from build123d import *

# Parameters (mm, degrees)
SKETCH1_W           = 54.8
SKETCH1_H           = 59.3
BOSS_EXTRUDE1_DEPTH = 3
FILLET1_R           = 2.2
SKETCH2_W           = 3
SKETCH2_H           = 15
CUT_EXTRUDE1_DEPTH  = 41.483113764
CUT_EXTRUDE2_DEPTH  = 1.5


with BuildPart() as part:
    # Sketch1 → Boss-Extrude1 (new body)
    with BuildSketch(Plane(origin=(0, 0, 0), x_dir=(1, 0, 0), z_dir=(0, 1, 0))):
        Rectangle(SKETCH1_W, SKETCH1_H)
    extrude(amount=BOSS_EXTRUDE1_DEPTH)

    # Fillet1
    fillet1_edges = [part.edges().sort_by_distance(p)[0] for p in [
        (27.4, 1.5, 29.65),
        (-27.4, 1.5, 29.65),
        (-27.4, 1.5, -29.65),
        (27.4, 1.5, -29.65),
    ]]
    fillet(fillet1_edges, radius=FILLET1_R)

    # Sketch2 → Cut-Extrude1 (cut, through all)
    with BuildSketch(Plane(origin=(0, 3, 0), x_dir=(1, 0, 0), z_dir=(0, 1, 0))):
        with Locations((-24.5, -8.5)):
            Rectangle(SKETCH2_W, SKETCH2_H)
    extrude(amount=-CUT_EXTRUDE1_DEPTH, mode=Mode.SUBTRACT)

    # Sketch2<3> → Cut-Extrude2 (cut)
    with BuildSketch(Plane(origin=(0, 3, 0), x_dir=(1, 0, 0), z_dir=(0, 1, 0))):
        Polygon((-26, -16), (-26, -26), (26, -26), (26, 2), (-26, 2), (-26, -1), (-23, -1), (-23, -16), align=None)
    extrude(amount=-CUT_EXTRUDE2_DEPTH, mode=Mode.SUBTRACT)


solid = part.part
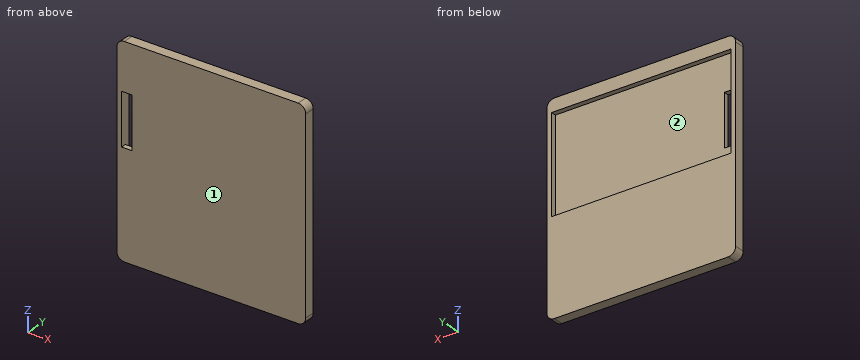
Input: part model. Units: mm. Frame: model coordinates. Face numbers are marked on the shaded views. Coordinates: 2 decimals unless noted, no trailing zeros. Loops run counter-clockwise (first coordinate to the right, second up) from the corner with the lowest first, then second, coordinate; pieces in that order, holes last. Notation, with made-up numbers: (-27.75, -35.75) -> (-16.75, -35.75) arc R21 cw to (-16.75, 0.25) -> close; hole circle Ø3 at (-33.5, 72.5). An arc over 180 degrees is marked (long way). Write item = value, one per line. Start each with the question number.
Item 1: Cut plane C-C, the plane x = -10.5. Return loops of the section in (y, z), plus the area to 3 significant figures.
Item 2: Cut plane B-B, the plane z = 9.5. Return loops of the section in (x, y), plus the area to 3 significant figures.
Item 3: Material intervals for line 1 (X direction, y = 1.75, z = 19); line 2 (X direction, y = 0.75, z = 10); line 3 (Z direction, x = -14, y = 1.7), sorted ascending.
Item 4: First-contact query: P1, Ø14, axis at x = 0.5, z = 9, coming from the +Y side. Flat tip, straight axial feed; report the tip coordinate or a pass-through.
Item 5: Cut plane A-A, the plane y = 2.05. Return loops of the section in (x, z), plus the area to 3 significant figures.
Item 6: Mould query, pull axis Z, two halves, no side actions, for the marked faces 1 and 2. Classes: pulls with the +Z half, pulls with the -Z half, needs draft (parallel to the pull), parting line crosses it, or undercut.
Ans:
q1.outline = (0, -29.65) -> (3, -29.65) -> (3, -2) -> (1.5, -2) -> (1.5, 26) -> (3, 26) -> (3, 29.65) -> (0, 29.65) -> close
q1.area = 136 mm²
q2.outline = (-27.4, 0) -> (-26, 0) -> (-26, 3) -> (-27.4, 3) -> close; (-23, 0) -> (27.4, 0) -> (27.4, 3) -> (26, 3) -> (26, 1.5) -> (-23, 1.5) -> close
q2.area = 81.9 mm²
q3.line_1 = -27.4 to -26, 26 to 27.4
q3.line_2 = -27.4 to -26, -23 to 27.4
q3.line_3 = -29.65 to -2, 26 to 29.65
q4.P1 = 1.5
q5.outline = (-27.4, -27.45) arc R2.2 ccw to (-25.2, -29.65) -> (25.2, -29.65) arc R2.2 ccw to (27.4, -27.45) -> (27.4, 27.45) arc R2.2 ccw to (25.2, 29.65) -> (-25.2, 29.65) arc R2.2 ccw to (-27.4, 27.45) -> close; hole (-26, -2) -> (26, -2) -> (26, 26) -> (-26, 26) -> close
q5.area = 1,790 mm²
q6.face_1 = needs draft
q6.face_2 = undercut
